Here's how the part is built. I have some questions about the finished solid (model axes, mm). Face numbers are marked on the shaded views. Give positions to 0.01 mm unless a question says otherwise; leave off trailing zeros. Loops run counter-clockwise (first coordinate to the right, second up) from the corner with the lowest first, then second, coordinate; pieces in that order, holes last.
Q1. If we section it at C-C (x = -0.5): Please give me the cut outline in (y, z).
Q2. If we section it at A-A (y = 2.45): Please give me the cut outline in (x, z), plus the area to 3 significant figures.
Q3. Will these pins go through, and if not, where does the flat tip stop? P1, Ø1.1, axis at y = 2.5, z = 1.5, coming from the -X side; P2, Ø2.5, axis at x = -8, z = 0.5, coming from the +Y side; P3, Ø0.5, axis at y = 2.5, z = -0.5, coming from the +X side.
Q4. If we section it at B-B (z = 0.5): Please give me the cut outline in (x, y).
Q5. I need wall thicknesses on line 1 (Y direction, x = -13.5, z = -3); line 2 (X direction, y = 2.55, z = -1.5); line 3 (X direction, y = 2.4, z = 3). Which ranges of each line are inside material? Lowest first, please.
Q6. We'd pull the mould along X, two halves only. Please class the marked faces 1, 2 and 3: +X half, -X half, draft (parallel to the pull), parting line (faces both ways), or undercut.
Q7. If we section it at D-D (y = 0.65): Please give me the cut outline in (x, z).
from build123d import *

# Parameters (mm, degrees)
BOSS_EXTRUDE1_DEPTH = 2
BOSS_EXTRUDE2_DEPTH = 1


with BuildPart() as part:
    # Sketch1 → Boss-Extrude1 (new body)
    with BuildSketch(Plane(origin=(0, 0, 0), x_dir=(1, 0, 0), z_dir=(0, 1, 0))):
        with BuildLine():
            Line((0, -4), (-26, -4))
            ThreePointArc((-26, -4), (-30, 0), (-26, 4))
            Line((-26, 4), (0, 4))
            ThreePointArc((0, 4), (4, 0), (0, -4))
        make_face()
    extrude(amount=BOSS_EXTRUDE1_DEPTH)

    # Sketch2 → Boss-Extrude2 (add)
    with BuildSketch(Plane(origin=(0, 2, 0), x_dir=(1, 0, 0), z_dir=(0, 1, 0))):
        with BuildLine():
            Line((-26, 4), (-26, -4))
            ThreePointArc((-26, -4), (-28.828427125, -2.828427125), (-30, 0))
            ThreePointArc((-30, 0), (-28.828427125, 2.828427125), (-26, 4))
        make_face()
        with BuildLine():
            Line((0, 4), (0, -4))
            ThreePointArc((0, -4), (4, 0), (0, 4))
        make_face()
    extrude(amount=BOSS_EXTRUDE2_DEPTH)


solid = part.part
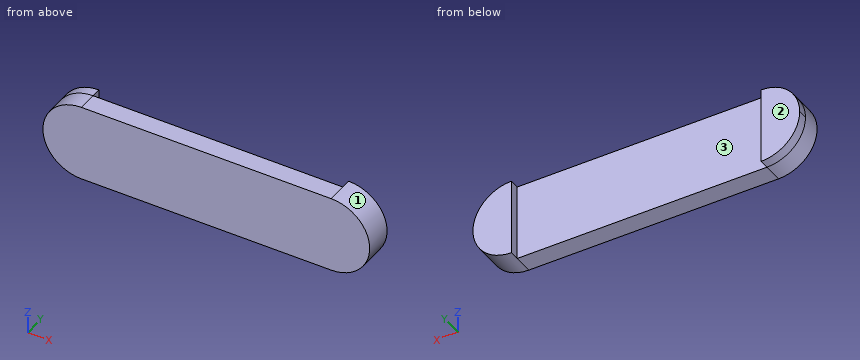
Check sheet entries:
1. outline: (0, -4) - (2, -4) - (2, 4) - (0, 4) - close
2. outline: (-26, -4) - (-26, 4) arc R4 ccw to start; (0, -4) arc R4 ccw to (0, 4) - close
2. area: 50.3 mm2
3. P1: stops at x = -29.89
3. P2: stops at y = 2
3. P3: stops at x = 3.99
4. outline: (-29.97, 0) - (3.97, 0) - (3.97, 3) - (0, 3) - (0, 2) - (-26, 2) - (-26, 3) - (-29.97, 3) - close
5. line 1: y = 0 to 2
5. line 2: x = -29.71 to -26, 0 to 3.71
5. line 3: x = -28.65 to -26, 0 to 2.65
6. face 1: +X half
6. face 2: draft
6. face 3: undercut
7. outline: (-26, -4) - (0, -4) arc R4 ccw to (0, 4) - (-26, 4) arc R4 ccw to start
